The figure shows three views and two pictorial views of one solid part (mm, origin at its lowest corner). Answer the questions. A direction names the side the tool comes from. Give positions to 0.01 mm unless a question says otherwise; leave off trailing zeros. Order: outer loops, then holes, each group sorted by start corner. A loop starts at its lowest first (then second) coordinate and runs counter-clockwise, first axis right, second up. Notation, with made-up numbers: M 51.5,70.5 L 86.5,70.5 A18 cw 86.5,78.5 Z; hole C -26.5,81 d2. An arc over 180 degrees is marked long. Write item = value, one per line. Start each with the question number.
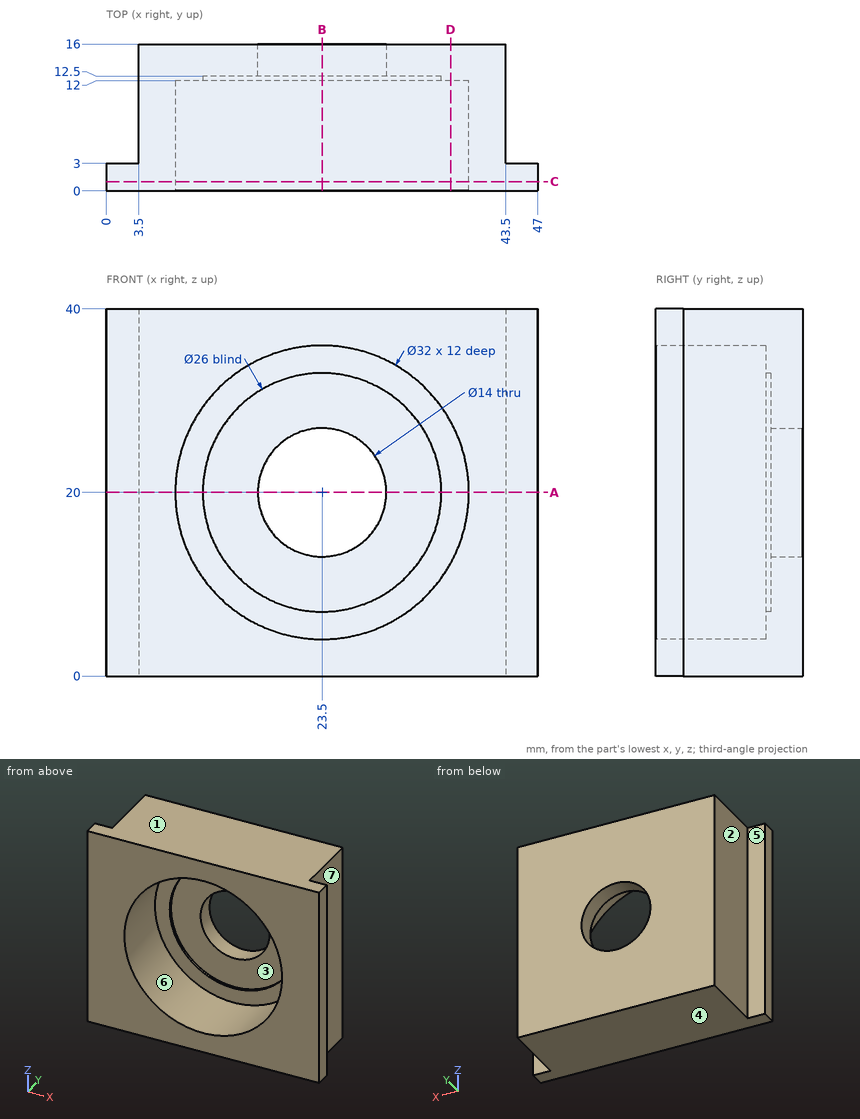
1) Find the intervals of material crossed by probe 1 along Z at (x, y) = (23.5, 13.55); probe 2 along Y at (x, z) = (45.5, 36.5); probe 3 along Z at (x, y) = (23.5, 12.2), in increasing order. Write a range as [from, to].
2) Find section C-C on y = 1. Determine the outline of the cut face in (x, z), plus the area to 3 significant figures.
3) For a pull along Z with two mould halves and no side action, classify the marked faces 1, 2, 3 and 4 as pulls with the +Z half, pulls with the -Z half, needs draft (parallel to the pull), parting line crosses it, or undercut.
4) For the marked faces 5, 6 and 7, determine the directions among +Z, -Z, +X, -X, +Y, -Y from which every point of the face is accessible in a straight line to the end or side of a thin tool.
5) Each of these flat-tipped pins is pushed along its axis until it touches: P1, Ø3, axis at y = 9.5, z = 9, coming from the +X side; P2, Ø1, axis at x = 2, z = 27, coming from the +Y side; P3, Ø8, axis at x = 28.5, z = 20, coming from the -Y side; P4, Ø8.5, axis at x = 23.5, z = 20, coming from the +Y side. Where does it stop, or does it pass through?
6) Find section D-D on x = 37.5. Determine the outline of the cut face in (y, z), plus the area to 3 significant figures.
7) Find section B-B on x = 23.5. Determine the outline of the cut face in (y, z).
8) Find section A-A on z = 20. Determine the outline of the cut face in (x, y), plus the area to 3 significant figures.
Numbers:
q1.probe_1 = [0, 13], [27, 40]
q1.probe_2 = [0, 3]
q1.probe_3 = [0, 7], [33, 40]
q2.outline = M 0,0 L 47,0 L 47,40 L 0,40 Z; hole C 23.5,20 d32
q2.area = 1,080 mm2
q3.face_1 = pulls with the +Z half
q3.face_2 = needs draft
q3.face_3 = undercut
q3.face_4 = pulls with the -Z half
q4.face_5 = +Z, -Z, -X, +Y
q4.face_6 = -Y
q4.face_7 = +Z, -Z, +X, +Y
q5.P1 = 43.5
q5.P2 = 3
q5.P3 = 12.5
q5.P4 = through
q6.outline = M 0,0 L 16,0 L 16,40 L 0,40 L 0,27.75 L 12,27.75 L 12,12.25 L 0,12.25 Z
q6.area = 454 mm2
q7.outline = M 0,0 L 16,0 L 16,13 L 12.5,13 L 12.5,7 L 12,7 L 12,4 L 0,4 Z; M 0,36 L 12,36 L 12,33 L 12.5,33 L 12.5,27 L 16,27 L 16,40 L 0,40 Z
q8.outline = M 0,0 L 7.5,0 L 7.5,12 L 10.5,12 L 10.5,12.5 L 16.5,12.5 L 16.5,16 L 3.5,16 L 3.5,3 L 0,3 Z; M 30.5,12.5 L 36.5,12.5 L 36.5,12 L 39.5,12 L 39.5,0 L 47,0 L 47,3 L 43.5,3 L 43.5,16 L 30.5,16 Z
q8.area = 215 mm2
